Autodesk Fusion 360 part; units mm, degrees
sketch "Sketch1" plane through (0, 0, 0) normal (0, 0, 1) x (1, 0, 0)
  line L0 (0, 0) -> (17, 0)
  line L1 (17, 0) -> (17, -3)
  line L2 (17, -3) -> (17, -5.7)
  line L3 (17, -5.7) -> (17, -12.3)
  line L4 (17, -12.3) -> (15, -12.3)
  line L5 (15, -12.3) -> (15, -0.8)
  line L6 (17, -3) -> (17, -4.35) construction
  line L7 (17, -4.35) -> (16.5, -4.35) construction
  line L8 (17, -3) -> (16.5, -4.35)
  line L9 (16.5, -4.35) -> (17, -5.7)
  line L10 (0, 0) -> (0, -0.8)
  line L11 (0, -0.8) -> (15, -0.8)
  dimension "d1" = 17
  dimension "d2" = 3
  dimension "d4" = 2.7
  dimension "d5" = 6.6
  dimension "d6" = 2
  dimension "d8" = 1.35
  dimension "d9" = 0.5
  dimension "d10" = 15
  dimension "d12" = 17
  dimension "d19" = 0.8
revolve "Revolve1" add sketch "Sketch1" angle 360 about axis through (0, 0, 0) along (0, -1, 0) contours L0 L1 L3 L4 L5 L8 L9 L10 L11
sketch "Sketch2" plane through (0, 0, 0) normal (0, 1, 0) x (-1, 0, 0)
  circle A0 centre (0, 0) radius 17
  circle A1 centre (0, 0) radius 16.575
  circle A2 centre (0, 0) radius 4.7
  dimension "d14" = 34
  dimension "d15" = 33.15
  dimension "d16" = 9.4
extrude "Extrude1" cut sketch "Sketch2" against normal blind 5 contours A2
equation "d15 = d14 - 0.85 mm"
Design review of the part built by this model. Coordinates are the model's own, in mm. A direction names the side the tool comes from. Coordinates: 2 decimals unless noted, no trailing zeros. Order: outer loops, then holes, each group sorted by start corner. A loop starts at its lowest first (then second) coordinate and runs counter-clockwise, first axis right, second up. Notation, with made-up numbers: (21.5, 28.25) -> (29.5, 28.25) arc R9 ccw to (29.5, 38.25) -> close; hole circle Ø6 at (51, 60.25). An arc over 180 degrees is marked (long way). One line per item, written item: value. Start each with the question number.
Q1. Take a section at A-A, the plane z = 0. State the section outline as (x, y) points, then the cut area to 3 significant figures.
Q2. Take a section at C-C, the plane y = -1.75. State the section outline as (x, z) points.
Q3. Take a section at B-B, the plane x = 0. State the section outline as (y, z) points.
Q4. Mouldability with a two-part tool opening along X and no side actions: class faces 3 (the cylindrical face through (9.139, -9.046, 14.334)), 4 (the cylindrical face through (1.02, -0.39, -4.59)), 5 (the flat face through (6, -12.3, -14)) as pulls with the +X half, pulls with the -X half, needs draft (parallel to the pull), parting line crosses it, or undercut.
Q5. For probe 1 along Z at (x, y) = (0, -6.25); probe 2 along Z at (x, y) = (0, -0.15); probe 3 along X at (y, z) = (-7.25, -1.5), list the stretches that pass through material, from the lowest coordinate up.
Q6. Tool access review of faces 1 (the cylindrical face through (9.139, -1.521, 14.334)), 2 (the cylindrical face through (-14.985, -6.47, -0.66)): name each direction out of +Z, -Z, +X, -X, +Y, -Y from which nothing blocks a thin tool from reaching the whole face with its end or side.
Q7. Insertion check: pin 1 Ø6 at (y, z) = (-3.5, 5.5) entering from +X; pin 2 Ø2 at (y, z) = (-10, 4.5) entering from -X; pin 3 Ø12 at (x, z) = (0, 0) entering from -Y. Each pin has a flat end and moves straight along its axis. Give the tip position at first contact, or say it passes through.
Values follow:
1. outline: (-17, -12.3) -> (-15, -12.3) -> (-15, -0.8) -> (-4.7, -0.8) -> (-4.7, 0) -> (-17, 0) -> (-17, -3) -> (-16.5, -4.35) -> (-17, -5.7) -> close; (4.7, -0.8) -> (15, -0.8) -> (15, -12.3) -> (17, -12.3) -> (17, -5.7) -> (16.5, -4.35) -> (17, -3) -> (17, 0) -> (4.7, 0) -> close
1. area: 64.3 mm2
2. outline: circle Ø34 at (0, 0); hole circle Ø30 at (0, 0)
3. outline: (-12.3, -17) -> (-5.7, -17) -> (-4.35, -16.5) -> (-3, -17) -> (0, -17) -> (0, -4.7) -> (-0.8, -4.7) -> (-0.8, -15) -> (-12.3, -15) -> close; (-12.3, 15) -> (-0.8, 15) -> (-0.8, 4.7) -> (0, 4.7) -> (0, 17) -> (-3, 17) -> (-4.35, 16.5) -> (-5.7, 17) -> (-12.3, 17) -> close
4. face 3: parting line crosses it
4. face 4: undercut
4. face 5: needs draft
5. probe 1: z = -17 to -15, 15 to 17
5. probe 2: z = -17 to -4.7, 4.7 to 17
5. probe 3: x = -16.93 to -14.92, 14.92 to 16.93
6. face 1: +Y, -Y
6. face 2: -Y
7. pin 1: stops at x = 16.81
7. pin 2: stops at x = -16.64
7. pin 3: stops at y = -0.8
